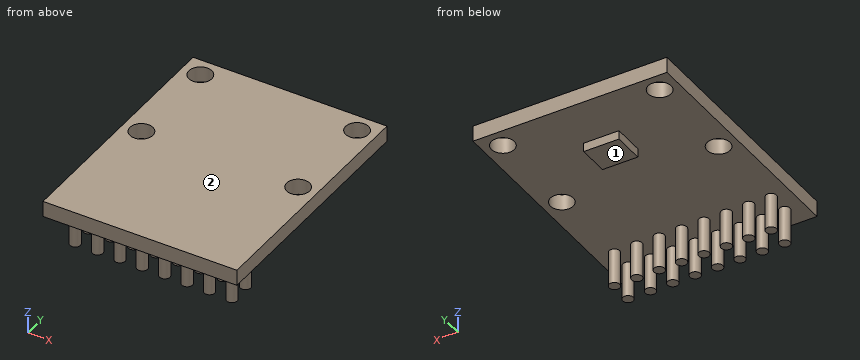
Autodesk Inventor part; units mm, degrees
ref_plane "YZ Plane" through (0, 0, 0) normal (1, 0, 0) x (0, 1, 0)
ref_plane "XZ Plane" through (0, 0, 0) normal (0, 1, 0) x (-1, 0, 0)
ref_plane "XY Plane" through (0, 0, 0) normal (0, 0, 1) x (1, 0, 0)
sketch "Skizze1" plane through (0, 0, 0) normal (0, 0, 1) x (1, 0, 0)
  line L0 (-11, 14) -> (11, 14)
  line L1 (11, 14) -> (11, -14)
  line L2 (11, -14) -> (-11, -14)
  line L3 (-11, -14) -> (-11, 14)
  line L4 (0, 19.6) -> (0, -19.6) construction
  line L5 (-15.4, 0) -> (15.4, 0) construction
  line L6 (-8.89, 0.89) -> (8.89, 0.89) construction
  line L7 (8.89, 0.89) -> (8.89, 11.89) construction
  line L8 (8.89, 11.89) -> (-8.89, 11.89) construction
  line L9 (-8.89, 11.89) -> (-8.89, 0.89) construction
  circle A0 centre (-8.89, 0.89) radius 1.3
  circle A1 centre (8.89, 0.89) radius 1.3
  circle A2 centre (8.89, 11.89) radius 1.3
  circle A3 centre (-8.89, 11.89) radius 1.3
  line L10 (-11, 14) -> (-8.89, 11.89) construction
  line L11 (-8.89, -11.46) -> (8.89, -11.46) construction
  line L12 (8.89, -11.46) -> (8.89, -8.92) construction
  line L13 (8.89, -8.92) -> (-8.89, -8.92) construction
  line L14 (-8.89, -8.92) -> (-8.89, -11.46) construction
  circle A4 centre (-8.89, -11.46) radius 0.6
  circle A5 centre (-6.35, -11.46) radius 0.6
  circle A6 centre (-3.81, -11.46) radius 0.6
  circle A7 centre (-1.27, -11.46) radius 0.6
  circle A8 centre (1.27, -11.46) radius 0.6
  circle A9 centre (3.81, -11.46) radius 0.6
  circle A10 centre (6.35, -11.46) radius 0.6
  circle A11 centre (8.89, -11.46) radius 0.6
  circle A12 centre (-8.89, -8.92) radius 0.6
  circle A13 centre (-6.35, -8.92) radius 0.6
  circle A14 centre (-3.81, -8.92) radius 0.6
  circle A15 centre (-1.27, -8.92) radius 0.6
  circle A16 centre (1.27, -8.92) radius 0.6
  circle A17 centre (3.81, -8.92) radius 0.6
  circle A18 centre (6.35, -8.92) radius 0.6
  circle A19 centre (8.89, -8.92) radius 0.6
  line L15 (-2, 4.64) -> (2, 4.64)
  line L16 (2, 4.64) -> (2, 8.14)
  line L17 (2, 8.14) -> (-2, 8.14)
  line L18 (-2, 8.14) -> (-2, 4.64)
  line L19 (-8.89, 0.89) -> (8.89, 11.89) construction
  line L20 (-8.89, 11.89) -> (8.89, 0.89) construction
  line L21 (-8.89, 6.39) -> (8.89, 6.39) construction
  point P0 (0, 0)
  point P1 (0, 6.39)
  dimension "d0" = 22
  dimension "d1" = 28
  dimension "d2" = 11
  dimension "d3" = 17.78
  dimension "d4" = 2.6
  dimension "d5" = 135
  dimension "d6" = 2.54
  dimension "d9" = 2.54
  dimension "d12" = 2.54
  dimension "d15" = 4
  dimension "d16" = 3.5
  dimension "d17" = 2.54
  dimension "d18" = 1.2
extrude "Extrusion1" add sketch "Skizze1" along normal blind 1.8 contours L0 L1 L2 L3 | A4 | A5 | A6 | A7 | A8 | A9 | A10 | A11 | A12 | A13 | A14 | A15 | A16 | A17 | A18 | A19 | L18 L17 L16 L15
extrude "Extrusion2" add sketch "Skizze1" against normal blind 4 from surface at 0 contours A4 | A5 | A6 | A7 | A8 | A9 | A10 | A11 | A12 | A13 | A14 | A15 | A16 | A17 | A18 | A19
extrude "Extrusion3" add sketch "Skizze1" against normal blind 1 from surface at 0 contours L18 L17 L16 L15
properties part number "AS5047D"
CAD build for the part. Positions are in the model's coordinates, mm. Face numbers are marked on the shaded views. A direction names the side the tool comes from. Round coordinates to 2 decimals unless told otherwise and drop trailing zeros. Order: outer loops, then holes, each group sorted by start corner. A loop starts at its lowest first (then second) coordinate and runs counter-clockwise, first axis right, second up. Notation, with made-up numbers: (82, -30) -> (96, -30) arc R12 ccw to (96, -20) -> close; hole circle Ø8 at (-30, 25). An arc over 180 degrees is marked (long way). Write each question's results on one line, items separated by ' | '.
1. Cut at D-D (z = 1.4). Give the cut face in (x, y), plus the area to 3 significant figures.
Findings below:
outline: (-11, -14) -> (11, -14) -> (11, 14) -> (-11, 14) -> close; hole circle Ø2.6 at (-8.89, 0.89); hole circle Ø2.6 at (-8.89, 11.89); hole circle Ø2.6 at (8.89, 0.89); hole circle Ø2.6 at (8.89, 11.89) | area: 595 mm²
2. Wall check: line 1 along Y through (x, z) = (8.89, 1.45); line 2 along Y through (x, z) = (0.25, -0.2); line 3 along Z through (x, y) = (0.75, -4.75). Give the ranges that are in metal, low to high. Write a range as [from, to].
Findings below:
line 1: y = [-14, -0.41], [2.19, 10.59], [13.19, 14] | line 2: y = [4.64, 8.14] | line 3: z = [0, 1.8]
3. 3-axis set-ups, long thin cutter, end or side, ignore diameter. For the marked faces 1 and 2: which of +Z, -Z, +X, -X, +Y, -Y reach the whole face in a straight line?
Findings below:
face 1: -Z, +X, -X, +Y | face 2: +Z, +X, -X, +Y, -Y
4. Flat gauge pins, fed straight in: P1, Ø1.8, axis at x = 0.5, y = 7, coming from the -Z side; P2, Ø2, axis at x = 4.5, y = -6.5, coming from the -Z side; P3, Ø0.8, axis at x = 0.5, z = -0.5, coming from the -Y side. Where does each tip first touch, or does it go through?
Findings below:
P1: stops at z = -1 | P2: stops at z = 0 | P3: stops at y = -11.93
5. Cut at B-B (x = -8.89). Give the cut face in (y, z).
Findings below:
outline: (-14, 0) -> (-12.06, 0) -> (-12.06, -4) -> (-10.86, -4) -> (-10.86, 0) -> (-9.52, 0) -> (-9.52, -4) -> (-8.32, -4) -> (-8.32, 0) -> (-0.41, 0) -> (-0.41, 1.8) -> (-14, 1.8) -> close; (2.19, 0) -> (10.59, 0) -> (10.59, 1.8) -> (2.19, 1.8) -> close; (13.19, 0) -> (14, 0) -> (14, 1.8) -> (13.19, 1.8) -> close
6. Cut at C-C (y = 0.89). Give the cut face in (x, z), plus the area to 3 significant figures.
Findings below:
outline: (-11, 0) -> (-10.19, 0) -> (-10.19, 1.8) -> (-11, 1.8) -> close; (-7.59, 0) -> (7.59, 0) -> (7.59, 1.8) -> (-7.59, 1.8) -> close; (10.19, 0) -> (11, 0) -> (11, 1.8) -> (10.19, 1.8) -> close | area: 30.2 mm²
7. Cut at A-A (z = -1.8). Count the separate pieces of the cut face and the enclosed holes in it, plus the area to 3 significant figures.
Findings below:
separate pieces: 16 | enclosed holes: 0 | area: 18.1 mm²
